Study the drawing (mm; zero at the part's minimum x, y, z) and answer. Coordinates: 2 decimals unless noted, no trailing zeros. Loops run counter-clockwise (first coordinate to the right, second up) from the corner with the lowest first, then second, coordinate; pieces in that order, holes last. Notation, with made-up numbers: (26.5, 82) -> (75.5, 82) arc R22 cw to (75.5, 93) -> close; hole circle Ø10 at (39, 31). An arc over 180 degrees is marked (long way). Answer in a Markdown table with one row per item.
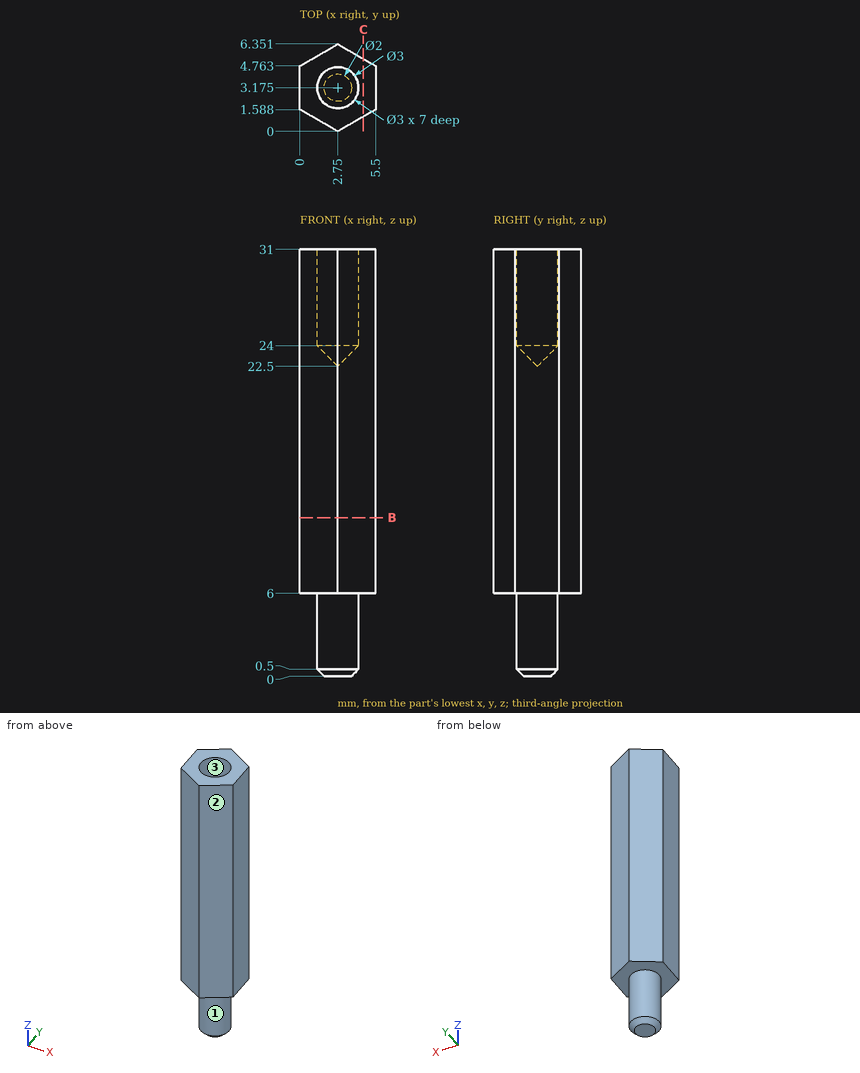
1. The mould has two halves that part along Y. Classify the marked faces 1, 2 and 3: pulls with the +Y half, pulls with the -Y half, needs draft (parallel to the pull), parting line crosses it, or undercut.
A:
| item | result |
|---|---|
| face 1 | parting line crosses it |
| face 2 | pulls with the -Y half |
| face 3 | undercut |
2. A cutting plane is placed at B-B on z = 11.5. Give the vertices of the cut face in (x, y).
A:
| item | result |
|---|---|
| outline | (0, 1.59) -> (2.75, 0) -> (5.5, 1.59) -> (5.5, 4.76) -> (2.75, 6.35) -> (0, 4.76) -> close |
3. Find the intervals of material crossed by probe 1 along Z at (x, y) = (4.3, 1.25); probe 2 along X at (y, z) = (3.5, 29) (1 decimal); probe 3 along X at (y, z) = (5.5, 11.5) (1 decimal), in increasing order.
A:
| item | result |
|---|---|
| probe 1 | z = 6 to 31 |
| probe 2 | x = 0 to 1.3, 4.2 to 5.5 |
| probe 3 | x = 1.3 to 4.2 |
4. Given pin 1 Ø2 at (x, z) = (4, 18) entering from -Y (1 decimal); pin 2 Ø2 at (x, z) = (4, 19) entering from +Y; pin 3 Ø1.6 at (x, y) = (2, 2) entering from -Z, each flat-ended and moving along its own axis, determine where each tip first touches the part or whether it passes through.
A:
| item | result |
|---|---|
| pin 1 | stops at y = 0.1 |
| pin 2 | stops at y = 6.21 |
| pin 3 | stops at z = 0 |
5. A cutting plane is placed at C-C on x = 4.6. Give the vertices of the cut face in (y, z).
A:
| item | result |
|---|---|
| outline | (1.07, 6) -> (5.28, 6) -> (5.28, 31) -> (1.07, 31) -> close |
